The model under review builds one solid part; all positions refer to its coordinate system, in mm. Face numbers are marked on the shaded views. A direction names the side the tool comes from. Round coordinates to 2 decimals unless told otherwise and drop trailing zeros. Order: outer loops, then holes, each group sorted by start corner. A loop starts at its lowest first (then second) coordinate and runs counter-clockwise, first axis right, second up.
from build123d import *

# Parameters (mm, degrees)
SKETCH_R        = 3.5
SKETCH_R_2      = 5
PAD_DEPTH       = 12.5
SKETCH001_R     = 5.4
POCKET_DEPTH    = 11
SKETCH002_R     = 13.25
POCKET001_DEPTH = 11.1
SKETCH003_R     = 17.5
SKETCH003_R_2   = 5
PAD001_DEPTH    = 15.5
SKETCH004_R     = 13.25
POCKET002_DEPTH = 11


with BuildPart() as part:
    # Sketch → Pad (new body)
    with BuildSketch(Plane.YZ):
        with BuildLine():
            Line((-18.91428, -44), (-60, -44))
            Line((-60, -44), (-60, 0))
            Line((-60, 0), (60, 0))
            Line((60, 0), (60, -44))
            Line((60, -44), (18.91428, -44))
            ThreePointArc((-18.91428, -44), (0, -57.5), (18.91428, -44))
        make_face()
        with Locations((-36, -21.5)):
            Circle(SKETCH_R, mode=Mode.SUBTRACT)
        with Locations((36, -21.5)):
            Circle(SKETCH_R, mode=Mode.SUBTRACT)
        with Locations((0, -37.5)):
            Circle(SKETCH_R_2, mode=Mode.SUBTRACT)
    extrude(amount=PAD_DEPTH)

    # Sketch001 → Pocket (cut)
    with BuildSketch(Plane.YZ.offset(12.5)):
        with Locations((-36, -21.5)):
            Circle(SKETCH001_R)
        with Locations((36, -21.5)):
            Circle(SKETCH001_R)
    extrude(amount=-POCKET_DEPTH, mode=Mode.SUBTRACT)

    # Sketch002 → Pocket001 (cut)
    with BuildSketch(Plane(origin=(0, 0, 0), x_dir=(0, 1, 0), z_dir=(-1, 0, 0))):
        with Locations((0, 37.5)):
            Circle(SKETCH002_R)
    extrude(amount=-POCKET001_DEPTH, mode=Mode.SUBTRACT)

    # Sketch003 → Pad001 (new body)
    with BuildSketch(Plane.YZ.offset(12.5)):
        with Locations((0, -37.5)):
            Circle(SKETCH003_R)
        with Locations((0, -37.5)):
            Circle(SKETCH003_R_2, mode=Mode.SUBTRACT)
    extrude(amount=PAD001_DEPTH)

    # Sketch004 → Pocket002 (cut)
    with BuildSketch(Plane.YZ.offset(28)):
        with Locations((0, -37.5)):
            Circle(SKETCH004_R)
    extrude(amount=-POCKET002_DEPTH, mode=Mode.SUBTRACT)


solid = part.part
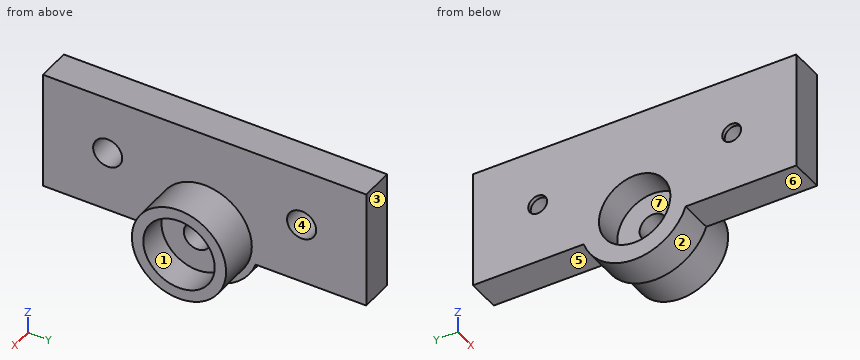
(1) Tool access review of the marked faces 5, 6 and 7: name each direction out of +Z, -Z, +X, -X, +Y, -Y from which nothing blocks a thin tool from reaching the whole face with its end or side.
(2) Clearance check with flat-ended pins moving along their axes: P1, Ø3, axis at y = -38.5, z = -19.5, coming from the +X side; P2, Ø6.5, axis at y = 36, z = -21.5, coming from the +X side; P3, Ø21, axis at y = -2, z = -39, coming from the +X side; P4, Ø3, axis at x = 5, y = -34.5, coming from the -Z side. State where each tip first meets the part, or that it passes through.
(3) We need section A-A (z = -37.5). Give the boundary of the cut face in (x, y), and give its area (3 significant figures).
(4) To check wall thickness, follow L1, parallel to Y at x = 0.45, z = -21.5; L2, parallel to Y at x = 7.25, z = -37.5; L3, parallel to Z at x = 10, y = 36. State the ranges of each line that lie inside material, in increasing order.
(5) We need section C-C (y = 0). Give the boundary of the cut face in (x, z), and give its area (3 significant figures).
(6) We need section D-D (z = -21.5). Give the boundary of the cut face in (x, y).
(7) We need section B-B (x = 8.75). Give the boundary of the cut face in (y, z), and give its area (3 significant figures).
(8) The part is to be moulded in two halves that separate along Z. For the marked faces 1, 2, 3 and 4, say which applies: pulls with the +Z half, pulls with the -Z half, needs draft (parallel to the pull), parting line crosses it, or undercut.
Verdict:
1. face 5: -Z, +X, -X, +Y
1. face 6: -Z, +X, -X, -Y
1. face 7: -X
2. P1: stops at x = 1.5
2. P2: passes through
2. P3: stops at x = 17
2. P4: stops at z = -44
3. outline: (0, -60) - (12.5, -60) - (12.5, -17.5) - (28, -17.5) - (28, -13.25) - (17, -13.25) - (17, -5) - (11.1, -5) - (11.1, -13.25) - (0, -13.25) - close; (0, 13.25) - (11.1, 13.25) - (11.1, 5) - (17, 5) - (17, 13.25) - (28, 13.25) - (28, 17.5) - (12.5, 17.5) - (12.5, 60) - (0, 60) - close
3. area: 1,400 mm2
4. L1: y = -60 to -39.5, -32.5 to 32.5, 39.5 to 60
4. L2: y = -60 to -13.25, 13.25 to 60
4. L3: z = -44 to -26.9, -16.1 to 0
5. outline: (0, -57.5) - (12.5, -57.5) - (12.5, -55) - (28, -55) - (28, -50.75) - (17, -50.75) - (17, -42.5) - (11.1, -42.5) - (11.1, -50.75) - (0, -50.75) - close; (0, -24.25) - (11.1, -24.25) - (11.1, -32.5) - (17, -32.5) - (17, -24.25) - (28, -24.25) - (28, -20) - (12.5, -20) - (12.5, 0) - (0, 0) - close
5. area: 617 mm2
6. outline: (0, -60) - (12.5, -60) - (12.5, -41.4) - (1.5, -41.4) - (1.5, -39.5) - (0, -39.5) - close; (0, -32.5) - (1.5, -32.5) - (1.5, -30.6) - (12.5, -30.6) - (12.5, -7.09) - (28, -7.09) - (28, 7.09) - (12.5, 7.09) - (12.5, 30.6) - (1.5, 30.6) - (1.5, 32.5) - (0, 32.5) - close; (0, 39.5) - (1.5, 39.5) - (1.5, 41.4) - (12.5, 41.4) - (12.5, 60) - (0, 60) - close
7. outline: (-60, -44) - (-18.91, -44) arc R20 ccw to (18.91, -44) - (60, -44) - (60, 0) - (-60, 0) - close; hole circle Ø10.8 at (-36, -21.5); hole circle Ø26.5 at (0, -37.5); hole circle Ø10.8 at (36, -21.5)
7. area: 4,920 mm2
8. face 1: undercut
8. face 2: pulls with the -Z half
8. face 3: needs draft
8. face 4: undercut
